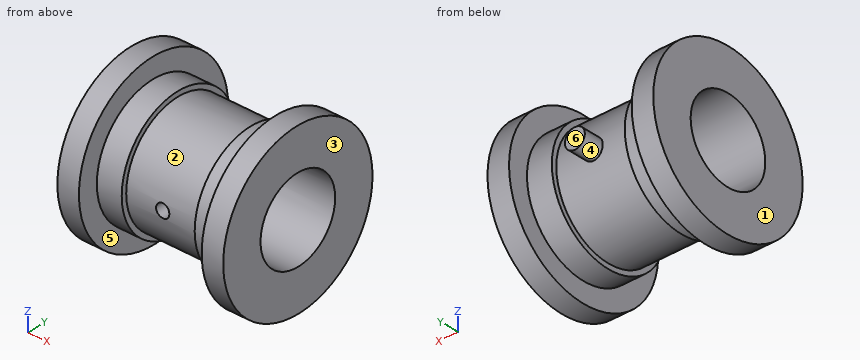
```python
from build123d import *

# Parameters (mm, degrees)
SKETCH2_R           = 2
CUT_EXTRUDE1_DEPTH  = 42
SKETCH3_R           = 3
BOSS_EXTRUDE1_DEPTH = 23.5
SKETCH20_R          = 12.5
CUT_EXTRUDE2_DEPTH  = 62.237243651


with BuildPart() as part:
    # Sketch1 → Revolve1 (revolve)
    with BuildSketch(Plane.XY):
        Polygon((25, 25), (25, 12.5), (-25, 12.5), (-25, 25), (-18.5, 25), (-18.5, 19), (-11, 19), (-11, 17.5), (11, 17.5), (11, 19), (18.5, 19), (18.5, 25), align=None)
    revolve(axis=Axis((25, 0, 0), (-1, 0, 0)))

    # Sketch2 → Cut-Extrude1 (cut)
    with BuildSketch(Plane(origin=(0, 0, 0), x_dir=(1, 0, 0), z_dir=(0, 1, 0))):
        with Locations(Location((0, 0, 0), (0, 0, 270))):
            Circle(SKETCH2_R)
    extrude(amount=-CUT_EXTRUDE1_DEPTH, mode=Mode.SUBTRACT)

    # Sketch3 → Boss-Extrude1 (add)
    with BuildSketch(Plane(origin=(0, 0, 0), x_dir=(1, 0, 0), z_dir=(0, 1, 0))):
        with Locations(Location((0, 0, 0), (0, 0, 180))):
            Circle(SKETCH3_R)
    extrude(amount=BOSS_EXTRUDE1_DEPTH)

    # Sketch20 → Cut-Extrude2 (cut, through all)
    with BuildSketch(Plane.ZY.offset(25)):
        with Locations(Location((0, 0, 0), (0, 0, 90))):
            Circle(SKETCH20_R)
    extrude(amount=-CUT_EXTRUDE2_DEPTH, mode=Mode.SUBTRACT)


solid = part.part
```
Can you work these out from the model? Positions are in its coordinate system, mm. Face numbers are marked on the shaded views. A direction names the side the tool comes from. Round coordinates to 2 decimals unless told otherwise and drop trailing zeros. Loops run counter-clockwise (first coordinate to the right, second up) from the corner with the lowest first, then second, coordinate; pieces in that order, holes last. Notation, with made-up numbers: M -26.5,72.5 L 22.5,72.5 A22 cw 22.5,93.5 Z; hole C -22.5,62 d9. An arc over 180 degrees is marked long. Write item = value, one per line. Start each with the question number.
(1) Suppose I cut it at A-A on z = 0. Give the number of separate pieces and of enclosed holes in the cut face, plus the area to 3 significant figures.
(2) I need wall thicknesses on line 1 along X through (y, z) = (4.5, -17.5); line 2 along Z through (x, y) = (-2, 0); line 3 along X through (y, z) = (11.5, 18). Which ranges of each line are inside material? Lowest first, please.
(3) Suppose I cut it at B-B on y = 0. Write out the boundary of the cut face in (x, z), plus the area to 3 significant figures.
(4) If we mould it in two halves opening along X, with no side actions, what happens to the marked faces 1, 2 and 3? For each: released by +X, released by -X, zero draft, split by the parting line, or undercut.
(5) I'm going to push flat-ended pins straight in: P1, Ø4.5, axis at x = 0, z = 0, coming from the +Y side; P2, Ø12, axis at x = 5.5, y = 0.5, coming from the +Z side; P3, Ø5, axis at x = 2.5, y = 2.5, coming from the -Z side. Where does each tip first touch, or does it pass through?
(6) Which directions (+Z, -Z, +X, -X, +Y, -Y) give clear straight access to the entire face, cutting with the end or side of a thin tool? Please do the marked faces 4, 5 and 6.
(7) Suppose I cut it at D-D on x = 21. Write out the boundary of the cut face in (y, z).
(8) Suppose I cut it at C-C on z = 22. Write out the boundary of the cut face in (x, y), plus the area to 3 significant figures.
Answer block:
q1.separate_pieces = 3
q1.enclosed_holes = 0
q1.area = 756 mm²
q2.line_1 = -25 to -11, 11 to 25
q2.line_2 = -17.5 to -12.5, 12.5 to 17.5
q2.line_3 = -25 to -18.5, 18.5 to 25
q3.outline = M -25,-25 L -18.5,-25 L -18.5,-19 L -11,-19 L -11,-17.5 L 11,-17.5 L 11,-19 L 18.5,-19 L 18.5,-25 L 25,-25 L 25,-12.5 L -25,-12.5 Z; M -25,12.5 L 25,12.5 L 25,25 L 18.5,25 L 18.5,19 L 11,19 L 11,17.5 L -11,17.5 L -11,19 L -18.5,19 L -18.5,25 L -25,25 Z
q3.area = 740 mm²
q4.face_1 = released by -X
q4.face_2 = undercut
q4.face_3 = released by +X
q5.P1 = 23.5
q5.P2 = 19
q5.P3 = -17.5
q6.face_4 = +Y
q6.face_5 = none
q6.face_6 = +Z, -Z, +Y
q7.outline = C 0,0 d50; hole C 0,0 d25
q8.outline = M -25,-11.87 L -18.5,-11.87 L -18.5,11.87 L -25,11.87 Z; M 18.5,-11.87 L 25,-11.87 L 25,11.87 L 18.5,11.87 Z
q8.area = 309 mm²
